Check sheet for the modelled part. Datum: model origin and axes. Units: mm. A direction names the side the tool comes from. Give positions to 0.01 mm unless a question says otherwise; leave off trailing zeros.
from build123d import *

# Parameters (mm, degrees)
SKETCH_1_R      = 3
SKETCH_1_W      = 2.8
SKETCH_1_H      = 5
SKETCH_1_W_2    = 2.85
EXTRUDE_1_DEPTH = 1.4


with BuildPart() as part:
    # Эскиз1 → Бобышка-Вытянуть1 (new, symmetric)
    with BuildSketch(Plane.XY):
        with BuildLine():
            ThreePointArc((175.091334091, 16.644787515), (168.620686799, 13.96455765), (165.940456932, 7.493910359))
            ThreePointArc((165.940456932, 7.493910359), (168.620686797, 1.023263065), (175.091334091, -1.656966802))
            add(Edge.make_bspline(
                [(175.091334091, -1.656966802), (177.330680613, -1.588466601), (181.854695323, -1.455127256), (188.663234462, -1.270383377), (195.516645168, -1.101112884), (202.369532894, -0.948617189), (211.49919029, -0.767742353), (220.603098666, -0.619939742), (229.617630172, -0.50292618), (236.087353854, -0.431514192), (241.980776913, -0.376520461), (246.558970011, -0.339535886), (249.120490965, -0.321271242), (250, -0.315)],
                knots=[0.704401069, 0.704401069, 0.704401069, 0.704401069, 0.730918775, 0.757971338, 0.785017763, 0.812061651, 0.839103366, 0.893099152, 0.919831065, 0.945809917, 0.969680601, 0.989589706, 1, 1, 1, 1], degree=3))
            ThreePointArc((250, -0.315), (250.130477272, 0), (250, 0.315))
            add(Edge.make_bspline(
                [(250, 0.315), (249.15566774, 0.545019818), (246.720175698, 1.208516243), (242.391332083, 2.358339053), (236.849761204, 3.787625364), (230.779918279, 5.298008837), (224.455917947, 6.812866028), (218.030543496, 8.291610632), (211.562405045, 9.719735057), (205.072411509, 11.092374932), (198.567970913, 12.407850726), (192.052369914, 13.665297924), (185.527619973, 14.864093303), (179.872800983, 15.850364437), (176.392239334, 16.431323122), (175.091334091, 16.644787515)],
                knots=[0, 0, 0, 0, 0.0101622, 0.029313053, 0.052011605, 0.076619468, 0.101948061, 0.127526132, 0.153184131, 0.178867888, 0.204557903, 0.230245712, 0.255925967, 0.281594302, 0.296903142, 0.296903142, 0.296903142, 0.296903142], degree=3))
        make_face()
        with Locations((175.091334091, 7.493910357)):
            Circle(SKETCH_1_R, mode=Mode.SUBTRACT)
        with Locations((188.091334091, 4.493910357)):
            Rectangle(SKETCH_1_W, SKETCH_1_H, mode=Mode.SUBTRACT)
        with Locations((205.091334091, 4.493910357)):
            Rectangle(SKETCH_1_W_2, SKETCH_1_H, mode=Mode.SUBTRACT)
    extrude(amount=EXTRUDE_1_DEPTH, both=True)


solid = part.part
1) Material ranges on L1, parallel to Y at x = 177, z = 1.1; L2, parallel to Y at x = 218, z = -0.1; L3, parallel to Y at x = 224, z = 0.05, recorded low to high.
Recorded:
L1: y = -1.6 to 5.18, 9.81 to 16.33
L2: y = -0.67 to 8.29
L3: y = -0.58 to 6.91
2) Depth check by flat-ended pin: pin 1 Ø0.8 at (x, z) = (188.5, -0.5) entering from -Y; pin 2 Ø9.5 at (x, y) = (175.09, 7.49) entering from +Z; pin 3 Ø1.4 at (x, z) = (204.5, 0.5) entering from +Y; pin 4 Ø0.8 at (y, z) = (4.5, 0) entering from -X. Enter the tip coordinate at first touch or a pass-through.
Recorded:
pin 1: stops at y = -1.29
pin 2: stops at z = 1.4
pin 3: stops at y = 11.34
pin 4: stops at x = 166.32
3) Draft check along X on faces 3 (the face through (198, 6, -1.4)), 4 (the face through (172.094, 7.626, -0.02)), 5 (the face through (165.943, 7.695, 0.02)). Enter one of: +X half, -X half, draft (parallel to the pull), parting line (faces both ways), or undercut.
Recorded:
face 3: draft
face 4: undercut
face 5: -X half
4) Set-up check for faces 1 (the face through (198, 6, 1.4)), 2 (the face through (205, 6.994, 0)): record each of +Z, -Z, +X, -X, +Y, -Y from which the full face is reachable in a straight line by a thin tool's end or side.
Recorded:
face 1: +Z, +X, -X, +Y, -Y
face 2: +Z, -Z
5) Section check A-A, the plane y = 5.5. State how many separate pieces and enclosed holes the cut face has, then the cut area to 3 significant figures.
Recorded:
separate pieces: 4
enclosed holes: 0
area: 150 mm2
